Input: part model. Units: mm. Frame: model coordinates. A direction names the side the tool comes from. Round coordinates to 2 decimals unless told otherwise and drop trailing zeros. Order: outer loops, then holes, each group sorted by start corner. A loop starts at its lowest first (then second) coordinate and runs counter-clockwise, first axis right, second up. Notation, with made-up numbers: (71.5, 11) -> (118.5, 11) arc R22 ccw to (118.5, 23) -> close; hole circle Ø7 at (52.25, 82.25). An arc over 180 degrees is marked (long way). Use a Markdown table: item, result.
from build123d import *

# Parameters (mm, degrees)
SKETCH1_R           = 23.5
SKETCH1_R_2         = 17.5
BOSS_EXTRUDE1_DEPTH = 6.93
SKETCH2_R           = 23
SKETCH2_R_2         = 22.5
CUT_EXTRUDE1_DEPTH  = 1
SKETCH3_R           = 19.5
SKETCH3_R_2         = 19
CUT_EXTRUDE2_DEPTH  = 1
FILLET1_R           = 0.2


with BuildPart() as part:
    # Sketch1 → Boss-Extrude1 (new body)
    with BuildSketch(Plane.XY):
        Circle(SKETCH1_R)
        Circle(SKETCH1_R_2, mode=Mode.SUBTRACT)
    extrude(amount=BOSS_EXTRUDE1_DEPTH)

    # Sketch2 → Cut-Extrude1 (cut)
    with BuildSketch(Plane.XY.offset(6.93)):
        Circle(SKETCH2_R)
        Circle(SKETCH2_R_2, mode=Mode.SUBTRACT)
    cut_extrude1 = extrude(amount=-CUT_EXTRUDE1_DEPTH, mode=Mode.SUBTRACT)

    # Sketch3 → Cut-Extrude2 (cut)
    with BuildSketch(Plane.XY.offset(6.93)):
        Circle(SKETCH3_R)
        Circle(SKETCH3_R_2, mode=Mode.SUBTRACT)
    cut_extrude2 = extrude(amount=-CUT_EXTRUDE2_DEPTH, mode=Mode.SUBTRACT)

    # Mirror1: Cut-Extrude1, Cut-Extrude2 across plane
    add(cut_extrude1.mirror(Plane.XY.offset(3.465)), mode=Mode.SUBTRACT)
    add(cut_extrude2.mirror(Plane.XY.offset(3.465)), mode=Mode.SUBTRACT)

    # Fillet1
    fillet1_edges = [part.edges().sort_by_distance(p)[0] for p in [
        (-22.5, 0, 6.93),
        (-19.5, 0, 6.93),
        (-22.5, 0, 0),
        (-19.5, 0, 0),
    ]]
    fillet(fillet1_edges, radius=FILLET1_R)


solid = part.part
1) Set-up query: faces 1 (the face through (18.7, -4.2, 5.93)), 2 (the face through (17, -15, 1)), 3 (the face through (0, -20, 0)). Return all of +Z, -Z, +X, -X, +Y, -Y with unobstructed straight access to the full face (end or side cutting, diameter ignored); none if empty.
Answer key:
| item | result |
|---|---|
| face 1 | +Z |
| face 2 | -Z |
| face 3 | -Z, +X, -X, +Y, -Y |
2) Contact query for flat-ended pins moving along their axis: P1, Ø1, axis at x = -1, z = 4, coming from the -Y side; P2, Ø1, axis at y = 14.5, z = 1.5, coming from the -X side; P3, Ø2, axis at x = -6, z = 6, coming from the +Y side; P4, Ø14, axis at x = 10, y = -2, coming from the -Z side. Output: stop coordinate, or through.
Answer key:
| item | result |
|---|---|
| P1 | stops at y = -23.49 |
| P2 | stops at x = -18.87 |
| P3 | stops at y = 22.96 |
| P4 | passes through |
3) Draft query along X for faces 4 (the face through (-13.887, -10.648, 3.416)), 5 (the face through (-2.994, 22.804, 6.437)), 6 (the face through (16, -17, 6.93)). Return one class per face: released by +X, released by -X, zero draft, split by the parting line, or undercut.
Answer key:
| item | result |
|---|---|
| face 4 | undercut |
| face 5 | undercut |
| face 6 | zero draft |
4) Ray query, probe 1 along Y at (x, z) = (0, 6.25); probe 2 along X at (y, z) = (-11, 0.75); probe 3 along Y at (x, z) = (12.5, 6). Return the intervals inside material, ascending.
Answer key:
| item | result |
|---|---|
| probe 1 | y = -23.5 to -23, -22.5 to -19.5, -19 to -17.5, 17.5 to 19, 19.5 to 22.5, 23 to 23.5 |
| probe 2 | x = -20.77 to -20.2, -19.63 to -16.1, -15.49 to -13.61, 13.61 to 15.49, 16.1 to 19.63, 20.2 to 20.77 |
| probe 3 | y = -19.9 to -19.31, -18.71 to -14.97, -14.31 to -12.25, 12.25 to 14.31, 14.97 to 18.71, 19.31 to 19.9 |
5) Cut plane A-A on z = 4. Return loops of the section in (x, y).
Answer key:
| item | result |
|---|---|
| outline | circle Ø47 at (0, 0); hole circle Ø35 at (0, 0) |
